Here's the drawing with two shaded views (mm, measured from the low corner). I have some questions. Give positions to 0.01 mm unless a question says otherwise; leave off trailing zeros. Write each loop counter-clockwise with the first axis right and the second up, starting at its lowest first coordinate (ties: lowest second). Pieces come first, ordered by that corner, then holes. Notation, with made-up numbers: (-38.75, 18.5) -> (-18.75, 18.5) arc R12 cw to (-18.75, 28.5) -> close; hole circle Ø7 at (33, -35.75). An arc over 180 degrees is marked (long way). Put each result on its own line as item: value. Start each with the question number.
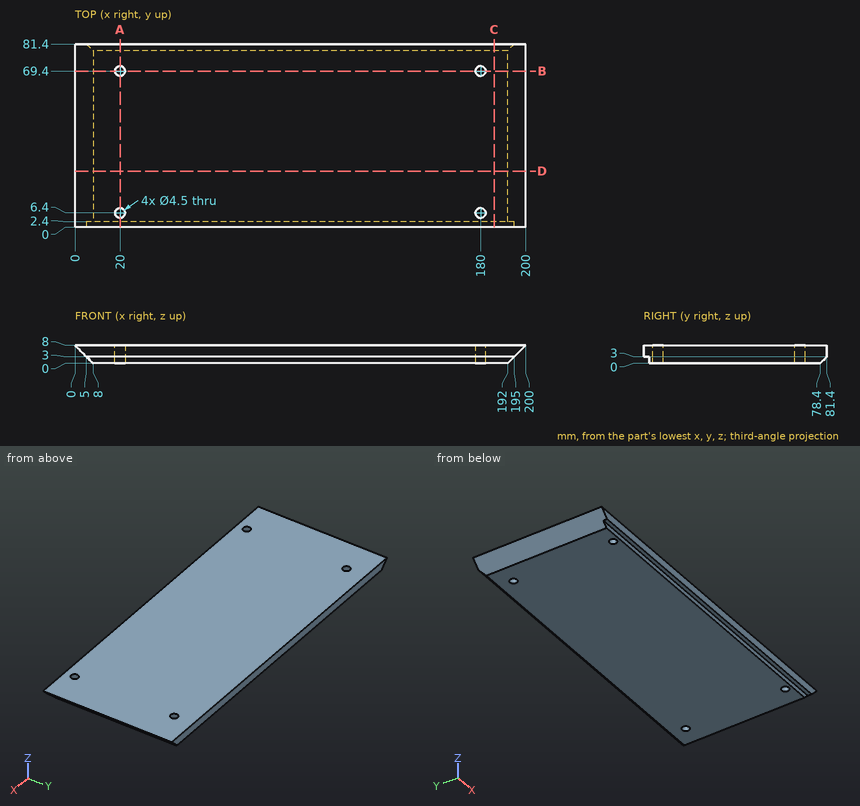
1) I want a section at B-B, the plane y = 69.4. Write out the boundary of the cut face in (x, z), and give its area (3 significant figures).
2) I want a section at D-D, the plane y = 25. Write out the boundary of the cut face in (x, z).
3) I need wall thicknesses on probe 1 along Y at (x, z) = (20, 4.25); probe 2 along Y at (x, z) = (180, 2.3); probe 3 along X at (y, z) = (68, 3.5). Which ranges of each line are inside material? Lowest first, please.
4) I'm going to push flat-ended pins straight in: pin 1 Ø4 at (x, y) = (20, 69.4) entering from -Z; pin 2 Ø1.9 at (x, y) = (78.5, 1) entering from -Z; pin 3 Ø1.5 at (x, z) = (163.5, 1) entering from +Y; pin 4 Ø3 at (y, z) = (31, 5.5) entering from +X. Where does each tip first touch, or does it pass through?
5) I want a section at A-A, the plane x = 20. Write out the boundary of the cut face in (y, z).
6) I want a section at C-C, the plane x = 186. Write out the boundary of the cut face in (y, z).
Established:
1. outline: (0, 8) -> (8, 0) -> (17.75, 0) -> (17.75, 8) -> close; (22.25, 0) -> (177.75, 0) -> (177.75, 8) -> (22.25, 8) -> close; (182.25, 0) -> (192, 0) -> (200, 8) -> (182.25, 8) -> close
1. area: 1,460 mm2
2. outline: (0, 8) -> (8, 0) -> (192, 0) -> (200, 8) -> close
3. probe 1: y = 0 to 4.15, 8.65 to 67.15, 71.65 to 81.4
3. probe 2: y = 2.4 to 4.15, 8.65 to 67.15, 71.65 to 80.7
3. probe 3: x = 4.5 to 18.24, 21.76 to 178.24, 181.76 to 195.5
4. pin 1: passes through
4. pin 2: stops at z = 3
4. pin 3: stops at y = 80.15
4. pin 4: stops at x = 199
5. outline: (0, 3) -> (2.4, 3) -> (2.4, 0) -> (4.15, 0) -> (4.15, 8) -> (0, 8) -> close; (8.65, 0) -> (67.15, 0) -> (67.15, 8) -> (8.65, 8) -> close; (71.65, 0) -> (78.4, 0) -> (81.4, 3) -> (81.4, 8) -> (71.65, 8) -> close
6. outline: (0, 3) -> (2.4, 3) -> (2.4, 0) -> (78.4, 0) -> (81.4, 3) -> (81.4, 8) -> (0, 8) -> close
